Read the model definition and answer for the solid it produces. Units are mm, in the model's axes. Face numbers are marked on the shaded views. Coordinates: 2 decimals unless noted, no trailing zeros. Loops run counter-clockwise (first coordinate to the right, second up) from the corner with the lowest first, then second, coordinate; pieces in that order, holes last. Notation, with made-up numbers: (50.5, -27) - (98.5, -27) arc R8 ccw to (98.5, -13) - close; hole circle Ø6 at (58.5, 1). An arc over 180 degrees is marked (long way). Use one line per item in the form item = value. Start each with the question number.
1) A cutting plane is placed at D-D (y = 0). Give the vertices of the cut face in (x, z), and give its area (3 significant figures).
2) A cutting plane is placed at B-B (z = -15). Give the vertices of the cut face in (x, y).
3) The mould has two halves that part along Y. Classify the marked faces 1, 2 and 3: released by +Y, released by -Y, zero draft, split by the parting line, or undercut.
4) A cutting plane is placed at A-A (y = -27.5). Give the vertices of the cut face in (x, z), and give its area (3 significant figures).
5) A cutting plane is placed at C-C (x = 83.5). Give the vertices of the cut face in (y, z).
6) Each of these flat-tipped pins is pushed along its axis until it touches: P1, Ø3, axis at x = 132, z = -7.5, coming from the +Y side; P2, Ø1.3, axis at x = 2.5, z = 1.5, coming from the +Y side; P3, Ø3, axis at y = -34.5, z = -40.5, coming from the +X side; P4, Ø0.8, axis at x = 80, z = 1.5, coming from the +Y side. Where does it stop, or does it pass through?
7) Consider line 1 (Y direction, x = 87, z = -1); line 2 (X direction, y = 33.5, z = -6); line 3 (Y direction, x = 131, z = -35.5). Determine where each line is inside the solid, lowest interval first.
from build123d import *

# Parameters (mm, degrees)
REVOLVE1_ANGLE      = 180
SKETCH4_W           = 2.54
SKETCH4_H           = 94.488
SKETCH4_W_2         = 76.2
SKETCH4_H_2         = 2.54
BOSS_EXTRUDE1_DEPTH = 2.54
CUT_EXTRUDE1_DEPTH  = 2.54


with BuildPart() as part:
    # Sketch1 → Revolve1 (revolve)
    with BuildSketch(Plane.XY):
        Polygon((0, 0), (0, 52.324), (152.4, 52.324), (152.4, 47.244), (5.08, 47.244), (5.08, 0), align=None)
    revolve(axis=Axis((5.08, 0, 0), (-1, 0, 0)), revolution_arc=REVOLVE1_ANGLE)

    # Sketch4 → Boss-Extrude1 (add)
    with BuildSketch(Plane.XY):
        with Locations((2.54, 0)):
            Rectangle(SKETCH4_W, SKETCH4_H)
        with Locations((76.2, 49.784)):
            Rectangle(SKETCH4_W_2, SKETCH4_H_2)
        with Locations((76.2, -49.784)):
            Rectangle(SKETCH4_W_2, SKETCH4_H_2)
    extrude(amount=BOSS_EXTRUDE1_DEPTH)

    # Sketch5 → Cut-Extrude1 (cut)
    with BuildSketch(Plane(origin=(152.4, 0, 0), x_dir=(0, 0, -1), z_dir=(1, 0, 0))):
        with BuildLine():
            Line((3.81, 51.054), (3.81, 48.514))
            ThreePointArc((3.81, 48.514), (48.663377359, 0), (3.81, -48.514))
            Line((3.81, -48.514), (3.81, -51.054))
            ThreePointArc((3.81, -51.054), (51.195966794, 0), (3.81, 51.054))
        make_face()
    extrude(amount=-CUT_EXTRUDE1_DEPTH, mode=Mode.SUBTRACT)


solid = part.part
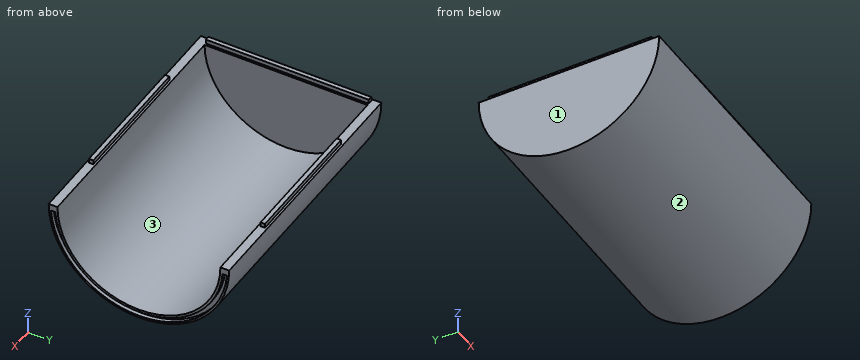
Found:
q1.outline = (0, -52.32) - (152.4, -52.32) - (152.4, -51.2) - (149.86, -51.2) - (149.86, -48.66) - (152.4, -48.66) - (152.4, -47.24) - (5.08, -47.24) - (5.08, 0) - (3.81, 0) - (3.81, 2.54) - (1.27, 2.54) - (1.27, 0) - (0, 0) - close
q1.area = 1,010 mm^2
q2.outline = (0, -50.13) - (152.4, -50.13) - (152.4, -48.95) - (149.86, -48.95) - (149.86, -46.29) - (152.4, -46.29) - (152.4, -44.8) - (5.08, -44.8) - (5.08, 44.8) - (152.4, 44.8) - (152.4, 46.29) - (149.86, 46.29) - (149.86, 48.95) - (152.4, 48.95) - (152.4, 50.13) - (0, 50.13) - close
q3.face_1 = zero draft
q3.face_2 = split by the parting line
q3.face_3 = undercut
q4.outline = (0, -44.51) - (152.4, -44.51) - (152.4, -43.18) - (149.86, -43.18) - (149.86, -40.15) - (152.4, -40.15) - (152.4, -38.42) - (5.08, -38.42) - (5.08, 0) - (3.81, 0) - (3.81, 2.54) - (1.27, 2.54) - (1.27, 0) - (0, 0) - close
q4.area = 1,120 mm^2
q5.outline = (-52.32, 0) arc R52.32 ccw to (52.32, 0) - (51.05, 0) - (51.05, 2.54) - (48.51, 2.54) - (48.51, 0) - (47.24, 0) arc R47.24 cw to (-47.24, 0) - (-48.51, 0) - (-48.51, 2.54) - (-51.05, 2.54) - (-51.05, 0) - close
q6.P1 = 51.98
q6.P2 = 47.24
q6.P3 = 152.4
q6.P4 = 51.05
q7.line_1 = -52.31 to -47.23, 47.23 to 52.31
q7.line_2 = 0 to 5.08
q7.line_3 = -38.44 to -31.17, 31.17 to 38.44
